from build123d import *

# Parameters (mm, degrees)
SKETCH_1_R      = 2.75
SKETCH_1_R_2    = 2.1
EXTRUDE_1_DEPTH = 3.4
SKETCH_1_3_R    = 4.6
SKETCH_1_3_R_2  = 2.75
SKETCH_1_3_R_3  = 2.1
EXTRUDE_2_DEPTH = 0.6


with BuildPart() as part:
    # Sketch 1 → Extrude 1 (new body)
    with BuildSketch(Plane(origin=(0, 0, 0), x_dir=(1, 0, 0), z_dir=(0, 1, 0))):
        Circle(SKETCH_1_R)
        Circle(SKETCH_1_R_2, mode=Mode.SUBTRACT)
    extrude(amount=EXTRUDE_1_DEPTH)

    # Sketch 1_3 → Extrude 2 (add)
    with BuildSketch(Plane(origin=(0, 0, 0), x_dir=(1, 0, 0), z_dir=(0, 1, 0))):
        Circle(SKETCH_1_3_R)
        Circle(SKETCH_1_3_R_2, mode=Mode.SUBTRACT)
        Circle(SKETCH_1_3_R_2)
        Circle(SKETCH_1_3_R_3, mode=Mode.SUBTRACT)
    extrude(amount=-EXTRUDE_2_DEPTH)


solid = part.part
Geometry: final body of the model. Coordinates: model frame, mm. A direction names the side the tool comes from. Coordinates: 2 decimals unless noted, no trailing zeros. Loops run counter-clockwise (first coordinate to the right, second up) from the corner with the lowest first, then second, coordinate; pieces in that order, holes last. Notation, with made-up numbers: (-24, 80.5) - (-9, 80.5) arc R25 ccw to (-9, 108.5) - close; hole circle Ø7 at (58.5, 62). An arc over 180 degrees is marked (long way). Put each result on its own line as item: value. Start each with the question number.
Q1. Pin query (flat end, axial travel): pin 1 Ø1 at (x, z) = (-2.5, -3) entering from +Y; pin 2 Ø2 at (y, z) = (0.5, -1.5) entering from +X; pin 3 Ø2 at (y, z) = (0.5, -3.5) entering from -X. Return the tip coordinate at first contact, or that it passes through.
Q2. Cut plane B-B, the plane x = 0. Return loops of the section in (y, z), and give its area (3 significant figures).
Q3. Set-up query: faces 1 (the flat face through (0, 0, 3)), 2 (the cylindrical face through (-3.65, -0.3, 2.8)). Return all of +Z, -Z, +X, -X, +Y, -Y with unobstructed straight access to the full face (end or side cutting, diameter ignored); none if empty.
Q4. Cut plane A-A, the plane z = 0. Return loops of the section in (x, y).
Q5. Line query: line 1 (Z direction, x = 0, y = -0.1); line 2 (Z direction, x = 0, y = 1.45). Output: solid intervals per line, ascending.
Q6. Cut plane D-D, the plane z = 2.25. Return loops of the section in (x, y), and give its area (3 significant figures).
Q7. Cut plane C-C, the plane y = 1.1. Return loops of the section in (x, z), and give its area (3 significant figures).
Filled sheet:
1. pin 1: y = 0
1. pin 2: x = 4.56
1. pin 3: x = -3.77
2. outline: (-0.6, -4.6) - (0, -4.6) - (0, -2.75) - (3.4, -2.75) - (3.4, -2.1) - (-0.6, -2.1) - close; (-0.6, 2.1) - (3.4, 2.1) - (3.4, 2.75) - (0, 2.75) - (0, 4.6) - (-0.6, 4.6) - close
2. area: 7.42 mm²
3. face 1: +Y
3. face 2: +Y, -Y
4. outline: (-4.6, -0.6) - (-2.1, -0.6) - (-2.1, 3.4) - (-2.75, 3.4) - (-2.75, 0) - (-4.6, 0) - close; (2.1, -0.6) - (4.6, -0.6) - (4.6, 0) - (2.75, 0) - (2.75, 3.4) - (2.1, 3.4) - close
5. line 1: -4.6 to -2.1, 2.1 to 4.6
5. line 2: -2.75 to -2.1, 2.1 to 2.75
6. outline: (-4.01, -0.6) - (4.01, -0.6) - (4.01, 0) - (1.58, 0) - (1.58, 3.4) - (-1.58, 3.4) - (-1.58, 0) - (-4.01, 0) - close
6. area: 15.6 mm²
7. outline: circle Ø5.5 at (0, 0); hole circle Ø4.2 at (0, 0)
7. area: 9.90 mm²
